Geometry: final body of the model. Coordinates: model frame, mm. Face numbers are marked on the shaded views. A direction names the side the tool comes from. Give positions to 0.01 mm unless a question says otherwise; leave off trailing zeros. Loops run counter-clockwise (first coordinate to the right, second up) from the corner with the lowest first, then second, coordinate; pieces in that order, holes last. Notation, with made-up numbers: M 44,-12 L 80,-12 A19 cw 80,2 Z; hole C -37,76.25 d1. An arc over 180 degrees is marked long. Put each result on its own line as item: value.
Autodesk Inventor part; units mm, degrees
ref_plane "YZ Plane" through (0, 0, 0) normal (1, 0, 0) x (0, 1, 0)
ref_plane "XZ Plane" through (0, 0, 0) normal (0, 1, 0) x (-1, 0, 0)
ref_plane "XY Plane" through (0, 0, 0) normal (0, 0, 1) x (1, 0, 0)
sketch "Sketch1" plane through (0, 0, 0) normal (0, 0, 1) x (1, 0, 0)
  line L0 (-12, 12) -> (12, 12)
  line L1 (12, 12) -> (12, -12)
  line L2 (12, -12) -> (-12, -12)
  line L3 (-12, -12) -> (-12, 12)
  line L4 (-12, 12) -> (12, -12) construction
  line L5 (12, 12) -> (-12, -12) construction
  point P0 (0, 0)
  dimension "d0" = 24
  dimension "d1" = 24
extrude "Extrusion1" add sketch "Sketch1" along normal blind 1
sketch "Sketch2" plane through (0, 0, 1) normal (0, 0, 1) x (1, 0, 0)
  line L0 (-10, 10) -> (10, 10)
  line L1 (10, 10) -> (10, -10)
  line L2 (10, -10) -> (-10, -10)
  line L3 (-10, -10) -> (-10, 10)
  line L4 (-10, 10) -> (10, -10) construction
  line L5 (10, 10) -> (-10, -10) construction
  point P0 (0, 0)
  dimension "d4" = 20
  dimension "d5" = 20
extrude "Extrusion2" add sketch "Sketch2" along normal blind 7
fillet "Fillet1" radius 4.1 8 edges at (10, 10, 4.5) (-10, 10, 4.5) (-10, -10, 4.5) (10, -10, 4.5) (12, -12, 0.5) (12, 12, 0.5) (-12, 12, 0.5) (-12, -12, 0.5)
chamfer "Chamfer1" distance 0.4 angle 45 8 edges at (-12, 0, 0) (-10.7991, -10.7991, 0) (0, -12, 0) (10.7991, -10.7991, 0) (12, 0, 0) (10.7991, 10.7991, 0) (0, 12, 0) (-10.7991, 10.7991, 0)
sketch "Sketch3" plane through (0, 0, 0) normal (0, 0, -1) x (-1, 0, 0)
  circle A0 centre (0, 0) radius 2.5
  circle A1 centre (7, 0) radius 2.5
  dimension "d12" = 5
  dimension "d15" = 7
extrude "Extrusion3" cut sketch "Sketch3" against normal through all
pattern_circular "Circular Pattern1" count 6 over 360 about axis through (0, 0, 0) along (0, 0, 1) of "Extrusion3"
equation "\"d1\" = d0"
properties part number "Speaker Cover"
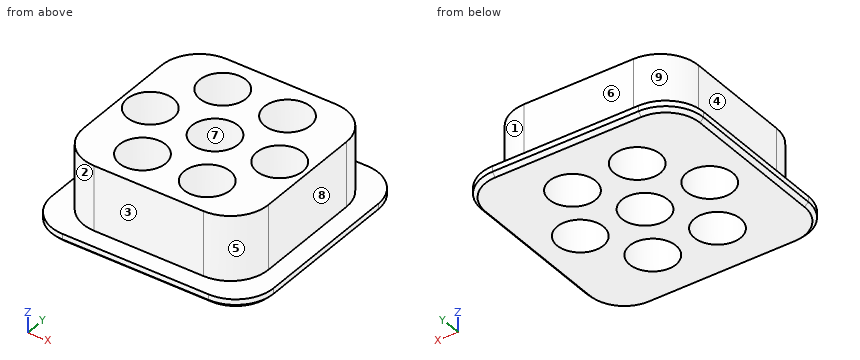
Item 1: Section C-C on y = -3. Output: boundary loops of the cut face in (x, z), then the cut area to 3 significant figures.
Output values:
outline: M -12,0.4 L -11.6,0 L 11.6,0 L 12,0.4 L 12,1 L 10,1 L 10,8 L -10,8 L -10,1 L -12,1 Z
area: 164 mm²
Item 2: Mould query, pull axis X, two halves, no side actions, for the marked faces 6, 7, 8 and 9. Classes: pulls with the +X half, pulls with the -X half, needs draft (parallel to the pull), parting line crosses it, or undercut.
Output values:
face 6: needs draft
face 7: undercut
face 8: pulls with the +X half
face 9: pulls with the -X half
Item 3: Line query: probe 1 along Y at (x, z) = (-3.5, 5); probe 2 along Y at (x, z) = (3.5, 0.5); probe 3 along Y at (x, z) = (0, 5.25). Output: solid intervals per line, ascending. Write a range as [from, to].
Output values:
probe 1: [-10, -8.56], [-3.56, 3.56], [8.56, 10]
probe 2: [-12, -8.56], [-3.56, 3.56], [8.56, 12]
probe 3: [-10, -2.5], [2.5, 10]
Item 4: Set-up query: the marked faces 1, 2, 3, 4 and 5. Return all of +Z, -Z, +X, -X, +Y, -Y with unobstructed straight access to the full face (end or side cutting, diameter ignored); none if empty.
Output values:
face 1: +Z, +X, +Y
face 2: +Z, -X, -Y
face 3: +Z, +X, -X, -Y
face 4: +Z, -X, +Y, -Y
face 5: +Z, +X, -Y
Item 5: Section B-B on y = 0. Output: boundary loops of the cut face in (x, z).
Output values:
outline: M -12,0.4 L -11.6,0 L -9.5,0 L -9.5,8 L -10,8 L -10,1 L -12,1 Z; M -4.5,0 L -2.5,0 L -2.5,8 L -4.5,8 Z; M 2.5,0 L 4.5,0 L 4.5,8 L 2.5,8 Z; M 9.5,0 L 11.6,0 L 12,0.4 L 12,1 L 10,1 L 10,8 L 9.5,8 Z
Item 6: Section D-D on z = 1.5. Output: boundary loops of the cut face in (x, y), then the cut area to 3 significant figures.
Output values:
outline: M -10,-5.9 A4.1 ccw -5.9,-10 L 5.9,-10 A4.1 ccw 10,-5.9 L 10,5.9 A4.1 ccw 5.9,10 L -5.9,10 A4.1 ccw -10,5.9 Z; hole C -7,0 d5; hole C -3.5,-6.06 d5; hole C -3.5,6.06 d5; hole C 0,0 d5; hole C 3.5,-6.06 d5; hole C 3.5,6.06 d5; hole C 7,0 d5
area: 248 mm²
Item 7: Pin query (flat end, axial travel): pin 1 Ø8 at (x, y) = (0, 0) entering from -Z; pin 2 Ø2 at (y, z) = (1, 6) entering from +X; pin 3 Ø1.5 at (x, z) = (-1.5, 4.5) entering from -Y; pin 4 Ø2 at (y, z) = (8, 5) entering from +X. Return the tip coordinate at first contact, or that it passes through.
Output values:
pin 1: z = 0
pin 2: x = 10
pin 3: y = -10
pin 4: x = 9.85
Item 8: Section A-A on x = 0. Output: boundary loops of the cut face in (y, z), then the cut area to 3 significant figures.
Output values:
outline: M -12,0.4 L -11.6,0 L -2.5,0 L -2.5,8 L -10,8 L -10,1 L -12,1 Z; M 2.5,0 L 11.6,0 L 12,0.4 L 12,1 L 10,1 L 10,8 L 2.5,8 Z
area: 124 mm²
